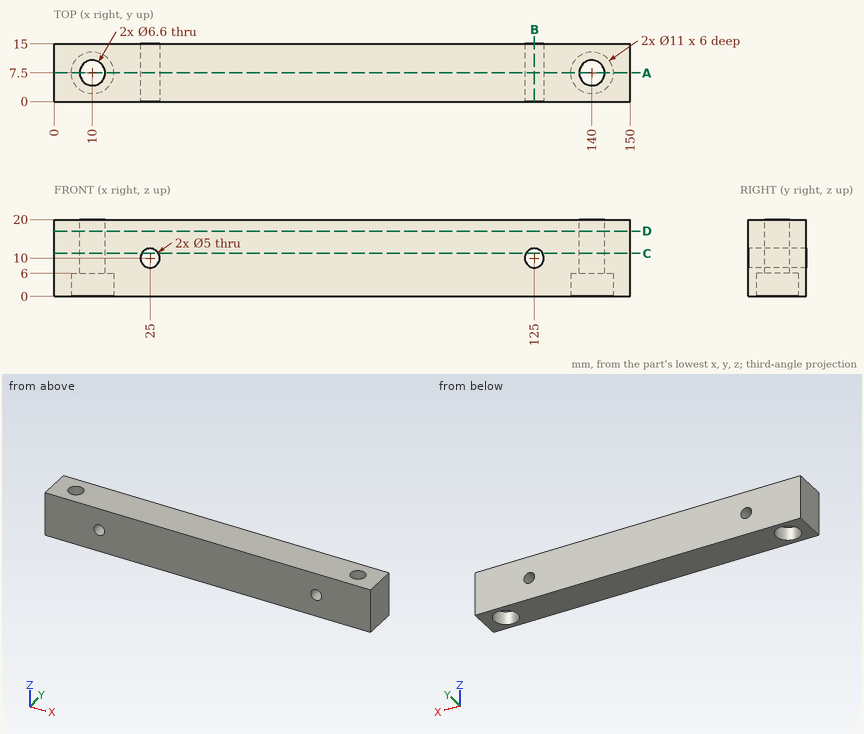
For this review, use the dimensioned drawing (mm, ordinates from the lowest corner) and the shaded views. Round coordinates to 2 decimals unless told otherwise and drop trailing zeros. Order: outer loops, then holes, each group sorted by start corner. A loop starts at its lowest first (then second) coordinate and runs counter-clockwise, first axis right, second up. Notation, with made-up numbers: M -39.75,79 L -24.75,79 A19 ccw -24.75,93 Z; hole C 66,88.25 d4. An arc over 180 degrees is marked long. Use a Markdown table: item, result. Add a question column.
Item 1: Insertion check: pin 1 (3.5 mm diameter, centred on x = 8, y = 8, fed in from -Z). The pin has a flat end and moves straight along its axis. Give the tip position at first contact, or say it passes through.
Item 2: Add section A-A, the plane y = 7.5. Give the boundary of the cut face in (x, z), then the cut area to 3 significant figures.
Item 3: To check wall thickness, follow line 1 along Z through (x, y) = (25, 9.25); line 2 along X through (y, z) = (6.5, 14.5); line 3 along Y through (x, z) = (10, 2.4). State the ranges of each line that lie inside material, in increasing order.
Item 4: Add section C-C, the plane z = 11.25. Give the boundary of the cut face in (x, y).
Item 5: Add section B-B, the plane x = 125. Give the boundary of the cut face in (y, z).
Item 6: Add section D-D, the plane z = 17. Give the boundary of the cut face in (x, y).
Geometry results:
| question | item | result |
|---|---|---|
| 1 | pin 1 | stops at z = 6 |
| 2 | outline | M 0,0 L 4.5,0 L 4.5,6 L 6.7,6 L 6.7,20 L 0,20 Z; M 13.3,6 L 15.5,6 L 15.5,0 L 134.5,0 L 134.5,6 L 136.7,6 L 136.7,20 L 13.3,20 Z; M 143.3,6 L 145.5,6 L 145.5,0 L 150,0 L 150,20 L 143.3,20 Z; hole C 25,10 d5; hole C 125,10 d5 |
| 2 | area | 2,640 mm² |
| 3 | line 1 | z = 0 to 7.5, 12.5 to 20 |
| 3 | line 2 | x = 0 to 6.86, 13.14 to 136.86, 143.14 to 150 |
| 3 | line 3 | y = 0 to 2, 13 to 15 |
| 4 | outline | M 0,0 L 22.83,0 L 22.83,15 L 0,15 Z; M 27.17,0 L 122.83,0 L 122.83,15 L 27.17,15 Z; M 127.17,0 L 150,0 L 150,15 L 127.17,15 Z; hole C 10,7.5 d6.6; hole C 140,7.5 d6.6 |
| 5 | outline | M 0,0 L 15,0 L 15,7.5 L 0,7.5 Z; M 0,12.5 L 15,12.5 L 15,20 L 0,20 Z |
| 6 | outline | M 0,0 L 150,0 L 150,15 L 0,15 Z; hole C 10,7.5 d6.6; hole C 140,7.5 d6.6 |
